For this review, take the finished solid that the model builds, in its own axes (mm). Face numbers are marked on the shaded views. A direction names the side the tool comes from. Round coordinates to 2 decimals unless told otherwise and drop trailing zeros. Loops run counter-clockwise (first coordinate to the right, second up) from the corner with the lowest first, then second, coordinate; pieces in that order, holes last. Notation, with made-up numbers: (59, -35) -> (75, -35) arc R31 cw to (75, -3) -> close; hole circle Ø5 at (1.25, 88). An arc over 180 degrees is marked (long way). Write each question's results on one line, items separated by ' | '.
```python
from build123d import *

# Parameters (mm, degrees)
SKETCH2_R           = 10
SKETCH2_R_2         = 3.5
BOSS_EXTRUDE1_DEPTH = 30
BOSS_EXTRUDE1_DRAFT = 1
SKETCH3_R           = 5.5
CUT_EXTRUDE1_DEPTH  = 22
CHAMFER1_SIZE       = 1
CHAMFER1_SIZE2      = 0.982994102
FILLET1_R           = 0.5
CUT_EXTRUDE2_DEPTH  = 27
CHAMFER2_SIZE       = 0.5
FILLET2_R           = 0.5


with BuildPart() as part:
    # Sketch2 → Boss-Extrude1 (with draft: the straight prism first)
    with BuildSketch(Plane(origin=(0, 0, 0), x_dir=(1, 0, 0), z_dir=(0, 1, 0))):
        Circle(SKETCH2_R)
        Circle(SKETCH2_R_2, mode=Mode.SUBTRACT)
    extrude(amount=BOSS_EXTRUDE1_DEPTH)
    # Boss-Extrude1: the draft: its side faces are tilted about the plane it starts from
    boss_extrude1_sides = [part.faces().sort_by_distance(p)[0] for p in [
        (-10, 15, 0),
        (-3.5, 15, 0),
    ]]
    draft(boss_extrude1_sides, Plane(origin=(0, 0, 0), x_dir=(1, 0, 0), z_dir=(0, 1, 0)), BOSS_EXTRUDE1_DRAFT)

    # Sketch3 → Cut-Extrude1 (cut)
    with BuildSketch(Plane(origin=(0, 30, 0), x_dir=(1, 0, 0), z_dir=(0, 1, 0))):
        with Locations(Location((0, 0, 0), (0, 0, 270))):
            Circle(SKETCH3_R)
    extrude(amount=-CUT_EXTRUDE1_DEPTH, mode=Mode.SUBTRACT)

    # Chamfer1
    chamfer1_edges = [part.edges().sort_by_distance(p)[0] for p in [
        (-3.5, 0, 0),
    ]]
    chamfer1_side = [part.faces().sort_by_distance(p)[0] for p in [
        (-3.56982026, 4, 0),
    ]]
    chamfer(chamfer1_edges, length=CHAMFER1_SIZE, length2=CHAMFER1_SIZE2, reference=chamfer1_side[0])

    # Fillet1
    fillet1_edges = [part.edges().sort_by_distance(p)[0] for p in [
        (-3.639640519, 8, 0),
    ]]
    fillet(fillet1_edges, radius=FILLET1_R)

    # Sketch4 → Cut-Extrude2 (cut)
    with BuildSketch(Plane.XZ):
        with BuildLine():
            Line((0, 3.5), (0, 10))
            ThreePointArc((0, 10), (0.261769483, 9.99657325), (0.523359562, 9.986295348))
            Line((0.523359562, 9.986295348), (0.183175847, 3.495203372))
            ThreePointArc((0.183175847, 3.495203372), (0.091619319, 3.498800637), (0, 3.5))
        make_face()
        with BuildLine():
            Line((3.031088913, 1.75), (8.660254038, 5))
            ThreePointArc((8.660254038, 5), (8.788171127, 4.771587603), (8.910065242, 4.539904997))
            Line((8.910065242, 4.539904997), (3.118522835, 1.588966749))
            ThreePointArc((3.118522835, 1.588966749), (3.075859894, 1.670055661), (3.031088913, 1.75))
        make_face()
        with BuildLine():
            Line((3.031088913, -1.75), (8.660254038, -5))
            ThreePointArc((8.660254038, -5), (8.526401644, -5.224985647), (8.386705679, -5.44639035))
            Line((8.386705679, -5.44639035), (2.935346988, -1.906236623))
            ThreePointArc((2.935346988, -1.906236623), (2.984240575, -1.828744977), (3.031088913, -1.75))
        make_face()
        with BuildLine():
            Line((0, -3.5), (0, -10))
            ThreePointArc((0, -10), (-0.261769483, -9.99657325), (-0.523359562, -9.986295348))
            Line((-0.523359562, -9.986295348), (-0.183175847, -3.495203372))
            ThreePointArc((-0.183175847, -3.495203372), (-0.091619319, -3.498800637), (0, -3.5))
        make_face()
        with BuildLine():
            Line((-3.031088913, -1.75), (-8.660254038, -5))
            ThreePointArc((-8.660254038, -5), (-8.788171127, -4.771587603), (-8.910065242, -4.539904997))
            Line((-8.910065242, -4.539904997), (-3.118522835, -1.588966749))
            ThreePointArc((-3.118522835, -1.588966749), (-3.075859894, -1.670055661), (-3.031088913, -1.75))
        make_face()
        with BuildLine():
            Line((-3.031088913, 1.75), (-8.660254038, 5))
            ThreePointArc((-8.660254038, 5), (-8.526401644, 5.224985647), (-8.386705679, 5.44639035))
            Line((-8.386705679, 5.44639035), (-2.935346988, 1.906236623))
            ThreePointArc((-2.935346988, 1.906236623), (-2.984240575, 1.828744977), (-3.031088913, 1.75))
        make_face()
    extrude(amount=-CUT_EXTRUDE2_DEPTH, mode=Mode.SUBTRACT)

    # Chamfer2
    chamfer2_edges = [part.edges().sort_by_distance(p)[0] for p in [
        (-0.378990673, 0, -7.231572831),
        (0, 0, -7.241497051),
        (-6.452221117, 0, -3.287570865),
        (-6.271320408, 0, -3.620748526),
        (-6.073230445, 0, 3.944001966),
        (-6.271320408, 0, 3.620748526),
        (0.378990673, 0, 7.231572831),
        (0, 0, 7.241497051),
        (6.452221117, 0, 3.287570865),
        (6.271320408, 0, 3.620748526),
        (6.073230445, 0, -3.944001966),
        (6.271320408, 0, -3.620748526),
    ]]
    chamfer(chamfer2_edges, length=CHAMFER2_SIZE)

    # Fillet2
    fillet2_edges = [part.edges().sort_by_distance(p)[0] for p in [
        (0, 30, -5.5),
    ]]
    fillet(fillet2_edges, radius=FILLET2_R)


solid = part.part
```
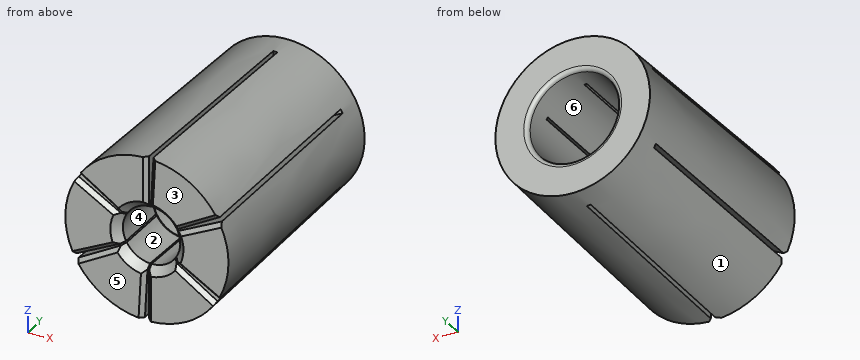
1. Consider section B-B (y = 15.5). State the section outline as (x, z) points, plus the area to 3 significant figures.
Values found:
outline: (-8.67, -4.42) -> (-4.9, -2.5) arc R5.5 cw to (-4.76, 2.75) -> (-8.43, 4.86) arc R9.73 ccw to start; (-8.43, -4.86) arc R9.73 ccw to (-0.51, -9.72) -> (-0.29, -5.49) arc R5.5 cw to (-4.76, -2.75) -> close; (-8.16, 5.3) -> (-4.61, 3) arc R5.5 cw to (0, 5.5) -> (0, 9.73) arc R9.73 ccw to start; (0, -9.73) arc R9.73 ccw to (8.16, -5.3) -> (4.61, -3) arc R5.5 cw to (0, -5.5) -> close; (0.29, 5.49) arc R5.5 cw to (4.76, 2.75) -> (8.43, 4.86) arc R9.73 ccw to (0.51, 9.72) -> close; (4.76, -2.75) -> (8.43, -4.86) arc R9.73 ccw to (8.67, 4.42) -> (4.9, 2.5) arc R5.5 cw to start | area: 192 mm2
2. Draft analysis for pull direction X (two halves, no side actions). For the marked faces 1, 2, 3 and 4, state which applies: released by +X, released by -X, zero draft, split by the parting line, or undercut.
Values found:
face 1: split by the parting line | face 2: undercut | face 3: zero draft | face 4: undercut
3. To check wall thickness, follow probe 1 along X at (y, z) = (12, 3.75); probe 2 along X at (y, z) = (13, 4.25); probe 3 along X at (y, z) = (12.75, 0). State the ranges of each line that lie inside material, in increasing order.
Values found:
probe 1: x = -9.04 to -6.5, -5.77 to -4.02, 4.02 to 6.5, 7.36 to 9.04 | probe 2: x = -8.8 to -7.36, -6.54 to -3.49, 3.49 to 7.36, 8.34 to 8.8 | probe 3: x = -9.78 to -5.5, 5.5 to 9.78
4. Tool access review of the marked faces 5 and 6: name each direction out of +Z, -Z, +X, -X, +Y, -Y from which nothing blocks a thin tool from reaching the whole face with its end or side.
Values found:
face 5: +Z, -Z, +X, -X, -Y | face 6: +Y
5. For pin 1 (6.5 mm diameter, centred on x = 0, z = 0, fed in from -Y); pin 2 (3 mm diameter, centred on y = 18, z = 4.5, fed in from -X); pin 3 (5 mm diameter, centred on y = 16.5, z = 7.5, fed in from +X); pin 4 (4 mm diameter, centred on x = -0.5, y = 14.5, fed in from -Z), all flat-tipped, find the tip position at first contact; note any pin that passes through.
Values found:
pin 1: passes through | pin 2: stops at x = -9.21 | pin 3: stops at x = 8.33 | pin 4: stops at z = -9.78
6. Consider section A-A (y = 5). State the section outline as (x, z) points.
Values found:
outline: (-8.83, -4.5) -> (-3.2, -1.63) arc R3.59 cw to (-3.11, 1.79) -> (-8.58, 4.96) arc R9.91 ccw to start; (-8.58, -4.96) arc R9.91 ccw to (-0.52, -9.9) -> (-0.19, -3.58) arc R3.59 cw to (-3.11, -1.79) -> close; (-8.31, 5.4) -> (-3.01, 1.95) arc R3.59 cw to (0, 3.59) -> (0, 9.91) arc R9.91 ccw to start; (0, -9.91) arc R9.91 ccw to (8.31, -5.4) -> (3.01, -1.95) arc R3.59 cw to (0, -3.59) -> close; (0.19, 3.58) arc R3.59 cw to (3.11, 1.79) -> (8.58, 4.96) arc R9.91 ccw to (0.52, 9.9) -> close; (3.11, -1.79) -> (8.58, -4.96) arc R9.91 ccw to (8.83, 4.5) -> (3.2, 1.63) arc R3.59 cw to start
